```python
from build123d import *

# Parameters (mm, degrees)
MAIN_BOARD_DEPTH    = 1.6
BOARD_HOLES_REACH   = 103.802
SKETCH3_R           = 1.375
MICROUSB_PWR_W      = 6.85
MICROUSB_PWR_H      = 5
USB_C_DEPTH         = 2.4
SKETCH5_W           = 6.4
SKETCH5_H           = 5.750421271
MICROHDMIS_DEPTH    = 3
SKETCH6_W           = 3
SKETCH6_H           = 22
CAMERA_PORT_DEPTH   = 5.5
SKETCH7_W           = 22
SKETCH7_H           = 16
ETHERNET_PORT_DEPTH = 13.5
SKETCH8_W           = 17.5
SKETCH8_H           = 15
USB_1_DEPTH         = 16
SKETCH9_W           = 17.5
SKETCH9_H           = 15
USB_2_DEPTH         = 16
SKETCH10_W          = 51
SKETCH10_H          = 5
GPIO_DEPTH          = 8.5
SKETCH11_W          = 6
SKETCH11_H          = 11.5
BOSS_EXTRUDE1_DEPTH = 1.125


with BuildPart() as part:
    # Sketch2 → Main Board (new body)
    with BuildSketch(Plane(origin=(0, 0, 0), x_dir=(1, 0, 0), z_dir=(0, 1, 0))):
        with BuildLine():
            Line((3, 0), (82, 0))
            ThreePointArc((82, 0), (84.121320344, 0.878679656), (85, 3))
            Line((85, 3), (85, 53))
            ThreePointArc((85, 53), (84.121320344, 55.121320344), (82, 56))
            Line((82, 56), (3, 56))
            ThreePointArc((3, 56), (0.878679656, 55.121320344), (0, 53))
            Line((0, 53), (0, 3))
            ThreePointArc((0, 3), (0.878679656, 0.878679656), (3, 0))
        make_face()
    extrude(amount=MAIN_BOARD_DEPTH)

    # Sketch3 → Board Holes (cut, up to next)
    with BuildSketch(Plane(origin=(0, 0, 0), x_dir=(1, 0, 0), z_dir=(0, 1, 0)), mode=Mode.PRIVATE) as board_holes_sk1:
        with Locations(Location((3.5, 3.5, 0), (0, 0, 90))):
            Circle(SKETCH3_R)
    board_holes_tool1 = extrude(board_holes_sk1.sketch, amount=BOARD_HOLES_REACH, mode=Mode.PRIVATE) & part.part
    # Sketch3 → Board Holes (cut, up to next)
    with BuildSketch(Plane(origin=(0, 0, 0), x_dir=(1, 0, 0), z_dir=(0, 1, 0)), mode=Mode.PRIVATE) as board_holes_sk2:
        with Locations(Location((3.5, 52.5, 0), (0, 0, 90))):
            Circle(SKETCH3_R)
    board_holes_tool2 = extrude(board_holes_sk2.sketch, amount=BOARD_HOLES_REACH, mode=Mode.PRIVATE) & part.part
    # Sketch3 → Board Holes (cut, up to next)
    with BuildSketch(Plane(origin=(0, 0, 0), x_dir=(1, 0, 0), z_dir=(0, 1, 0)), mode=Mode.PRIVATE) as board_holes_sk3:
        with Locations(Location((61.5, 52.5, 0), (0, 0, 90))):
            Circle(SKETCH3_R)
    board_holes_tool3 = extrude(board_holes_sk3.sketch, amount=BOARD_HOLES_REACH, mode=Mode.PRIVATE) & part.part
    # Sketch3 → Board Holes (cut, up to next)
    with BuildSketch(Plane(origin=(0, 0, 0), x_dir=(1, 0, 0), z_dir=(0, 1, 0)), mode=Mode.PRIVATE) as board_holes_sk4:
        with Locations(Location((61.5, 3.5, 0), (0, 0, 90))):
            Circle(SKETCH3_R)
    board_holes_tool4 = extrude(board_holes_sk4.sketch, amount=BOARD_HOLES_REACH, mode=Mode.PRIVATE) & part.part
    add(board_holes_tool1.solids().sort_by_distance((3.5, 0, -3.5))[0], mode=Mode.SUBTRACT)
    add(board_holes_tool2.solids().sort_by_distance((3.5, 0, -52.5))[0], mode=Mode.SUBTRACT)
    add(board_holes_tool3.solids().sort_by_distance((61.5, 0, -52.5))[0], mode=Mode.SUBTRACT)
    add(board_holes_tool4.solids().sort_by_distance((61.5, 0, -3.5))[0], mode=Mode.SUBTRACT)

    # MicroUSB PWR → USB C (add)
    with BuildSketch(Plane(origin=(0, 1.6, 0), x_dir=(1, 0, 0), z_dir=(0, 1, 0))):
        with Locations((11.2, 2)):
            Rectangle(MICROUSB_PWR_W, MICROUSB_PWR_H)
    extrude(amount=USB_C_DEPTH)

    # Sketch5 → MicroHDMIs (add)
    with BuildSketch(Plane(origin=(0, 1.6, 0), x_dir=(1, 0, 0), z_dir=(0, 1, 0))):
        with Locations((26, 2.375210636)):
            Rectangle(SKETCH5_W, SKETCH5_H)
        with Locations((39.5, 2.375210636)):
            Rectangle(SKETCH5_W, SKETCH5_H)
    extrude(amount=MICROHDMIS_DEPTH)

    # Sketch6 → Camera Port (add)
    with BuildSketch(Plane(origin=(0, 1.6, 0), x_dir=(1, 0, 0), z_dir=(0, 1, 0))):
        with Locations((46.5, 11.5)):
            Rectangle(SKETCH6_W, SKETCH6_H)
    extrude(amount=CAMERA_PORT_DEPTH)

    # Sketch7 → Ethernet port (add)
    with BuildSketch(Plane(origin=(0, 1.6, 0), x_dir=(1, 0, 0), z_dir=(0, 1, 0))):
        with Locations((76, 45.75)):
            Rectangle(SKETCH7_W, SKETCH7_H)
    extrude(amount=ETHERNET_PORT_DEPTH)

    # Sketch8 → USB 1 (add)
    with BuildSketch(Plane(origin=(0, 1.6, 0), x_dir=(1, 0, 0), z_dir=(0, 1, 0))):
        with Locations((78.25, 9)):
            Rectangle(SKETCH8_W, SKETCH8_H)
    extrude(amount=USB_1_DEPTH)

    # Sketch9 → USB 2 (add)
    with BuildSketch(Plane(origin=(0, 1.6, 1.6), x_dir=(1, 0, 0), z_dir=(0, 1, 0))):
        with Locations((78.25, 28.6)):
            Rectangle(SKETCH9_W, SKETCH9_H)
    extrude(amount=USB_2_DEPTH)

    # Sketch10 → GPIO (add)
    with BuildSketch(Plane(origin=(0, 1.6, 0), x_dir=(1, 0, 0), z_dir=(0, 1, 0))):
        with Locations((32.5, 52.5)):
            Rectangle(SKETCH10_W, SKETCH10_H)
    extrude(amount=GPIO_DEPTH)

    # Sketch11 → Boss-Extrude1 (add)
    with BuildSketch(Plane.XZ):
        with Locations((9, -28)):
            Rectangle(SKETCH11_W, SKETCH11_H)
    extrude(amount=BOSS_EXTRUDE1_DEPTH)


solid = part.part
```
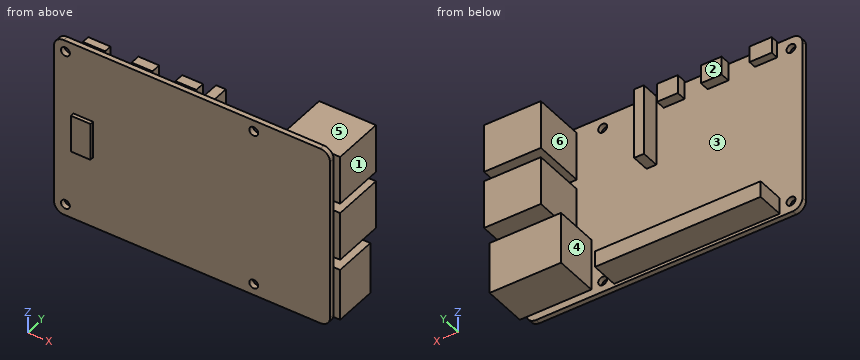
Input: part model. Units: mm. Frame: model coordinates. Face numbers are marked on the shaded views. A direction names the side the tool comes from. Coordinates: 2 decimals unless noted, no trailing zeros. Write each loop counter-clockwise with the first axis right and the second up, starting at its lowest first coordinate (ties: lowest second). Pieces come first, ordered by that corner, then holes. Notation, with made-up numbers: (9.5, 56.25) -> (43.5, 56.25) arc R32 cw to (43.5, 95.25) -> close; hole circle Ø3 at (83.5, -22). An arc over 180 degrees is marked (long way). Answer as a JSON object with one key per item and string values.
1. Section A-A on z = -32. Return the cut outline in (x, y) (3 decimals).
Result set:
{"outline": "(0, 0) -> (6, 0) -> (6, -1.125) -> (12, -1.125) -> (12, 0) -> (85, 0) -> (85, 1.6) -> (87, 1.6) -> (87, 17.6) -> (69.5, 17.6) -> (69.5, 1.6) -> (0, 1.6) -> close"}
2. Section B-B on x = 61.5. Return the cut outline in (y, z) (3 decimals).
Result set:
{"outline": "(0, -56) -> (1.6, -56) -> (1.6, -53.875) -> (0, -53.875) -> close; (0, -51.125) -> (1.6, -51.125) -> (1.6, -4.875) -> (0, -4.875) -> close; (0, -2.125) -> (1.6, -2.125) -> (1.6, 0) -> (0, 0) -> close"}
3. Section C-C on x = 26. Return the cut outline in (y, z).
Result set:
{"outline": "(0, -56) -> (1.6, -56) -> (1.6, -55) -> (10.1, -55) -> (10.1, -50) -> (1.6, -50) -> (1.6, -5.25) -> (4.6, -5.25) -> (4.6, 0.5) -> (1.6, 0.5) -> (1.6, 0) -> (0, 0) -> close"}
4. First-contact query: P1, Ø4.5, axis at x = 27.5, z = -2, coming from the +Y side; P2, Ø9.5, axis at x = 37.5, y = 6.5, coming from the -Z side; P3, Ø7, axis at y = 11.5, z = -42, coming from the -X side. Flat tips, straight axial feed; report the tip coordinate or a pass-through.
Result set:
{"P1": "stops at y = 4.6", "P2": "stops at z = -55", "P3": "stops at x = 65"}
5. Material intervals for line 1 (X direction, y = 1.2, z = -52.5) (3 decimals); line 2 (Z direction, x = 61.5, y = 0.4) (3 decimals); line 3 (Z direction, x = 37.5, y = 2), sorted ascending. Write a range as from..to.
Result set:
{"line 1": "x = 0..2.125, 4.875..60.125, 62.875..85", "line 2": "z = -56..-53.875, -51.125..-4.875, -2.125..0", "line 3": "z = -55..-50, -5.25..0.5"}
6. Section D-D on z = -17.5. Return the cut outline in (x, y), then the cut area to 4 significant figures.
Result set:
{"outline": "(0, 0) -> (85, 0) -> (85, 1.6) -> (48, 1.6) -> (48, 7.1) -> (45, 7.1) -> (45, 1.6) -> (0, 1.6) -> close", "area": "152.5 mm2"}
7. Mould query, pull axis X, two halves, no side actions, for the marked faces 1, 2 and 3. Classes: released by +X, released by -X, zero draft, split by the parting line, or undercut.
Result set:
{"face 1": "released by +X", "face 2": "zero draft", "face 3": "undercut"}
8. Access query for the marked faces 4, 5 and 6. Directions: +Z, -Z, +X, -X, +Y, -Y. A direction counts if a zero-diameter tool reaches every point of the face in a straight line with its end or side. Return the directions, or none.
Result set:
{"face 4": "+Z, -Z, +Y", "face 5": "+Z, +X, +Y", "face 6": "+Z, +Y"}
